Design review of the part built by this model. Coordinates are the model's own, in mm. A direction names the side the tool comes from. Round coordinates to 2 decimals unless told otherwise and drop trailing zeros. Order: outer loops, then holes, each group sorted by start corner. A loop starts at its lowest first (then second) coordinate and runs counter-clockwise, first axis right, second up. Notation, with made-up numbers: M 79,-27 L 90,-27 A22 cw 90,0 Z; hole C 3.5,20.25 d7. An arc over 180 degrees is marked long. Write item = value, one per line. Start each with the question number.
```python
from build123d import *

# Parameters (mm, degrees)
SKETCH2_R            = 15.24
BOSS_EXTRUDE1_DEPTH  = 5.08
SKETCH3_R            = 12.7
BOSS_EXTRUDE4_DEPTH  = 8.89
SKETCH4_R            = 7.62
SKETCH4_R_2          = 6.35
CUT_EXTRUDE2_DEPTH   = 0.508
SKETCH7_R            = 10.16
BOSS_EXTRUDE7_DEPTH  = 10.16
SKETCH8_R            = 6.35
SKETCH8_R_2          = 5.08
CUT_EXTRUDE6_DEPTH   = 1.27
SKETCH11_R           = 2.33542976
BOSS_EXTRUDE8_DEPTH  = 82.55
SKETCH12_R           = 6.35
BOSS_EXTRUDE9_DEPTH  = 2.54
SKETCH13_R           = 5.715
BOSS_EXTRUDE13_DEPTH = 1.905


with BuildPart() as part:
    # Sketch2 → Boss-Extrude1 (new body)
    with BuildSketch(Plane(origin=(0, 0, 0), x_dir=(1, 0, 0), z_dir=(0, 1, 0))):
        Circle(SKETCH2_R)
    extrude(amount=BOSS_EXTRUDE1_DEPTH)

    # Sketch3 → Boss-Extrude4 (add)
    with BuildSketch(Plane(origin=(0, 5.08, 0), x_dir=(1, 0, 0), z_dir=(0, 1, 0))):
        Circle(SKETCH3_R)
    extrude(amount=BOSS_EXTRUDE4_DEPTH)

    # Sketch4 → Cut-Extrude2 (cut)
    with BuildSketch(Plane(origin=(0, 13.97, 0), x_dir=(1, 0, 0), z_dir=(0, 1, 0))):
        Circle(SKETCH4_R)
        Circle(SKETCH4_R_2, mode=Mode.SUBTRACT)
    extrude(amount=-CUT_EXTRUDE2_DEPTH, mode=Mode.SUBTRACT)



with BuildPart() as body_2:
    # Sketch7 → Boss-Extrude7 (new body)
    with BuildSketch(Plane(origin=(0, 0, 0), x_dir=(1, 0, 0), z_dir=(0, 1, 0))):
        with Locations((0, -88.9)):
            Circle(SKETCH7_R)
    extrude(amount=BOSS_EXTRUDE7_DEPTH)

    # Sketch8 → Cut-Extrude6 (cut)
    with BuildSketch(Plane(origin=(0, 10.16, 0), x_dir=(1, 0, 0), z_dir=(0, 1, 0))):
        with Locations((0, -88.9)):
            Circle(SKETCH8_R)
        with Locations((0, -88.9)):
            Circle(SKETCH8_R_2, mode=Mode.SUBTRACT)
    extrude(amount=-CUT_EXTRUDE6_DEPTH, mode=Mode.SUBTRACT)


with BuildPart() as part_1:
    add(part.part)

    add(body_2.part)  # Boss-Extrude8 merges body 2
    # Sketch11 → Boss-Extrude8 (add)
    with BuildSketch(Plane.XY):
        with Locations((0, 2.324561436)):
            Circle(SKETCH11_R)
    extrude(amount=BOSS_EXTRUDE8_DEPTH)

    # Sketch12 → Boss-Extrude9 (add)
    with BuildSketch(Plane.XZ):
        with Locations((-0.225047318, 0)):
            Circle(SKETCH12_R)
    extrude(amount=BOSS_EXTRUDE9_DEPTH)

    # Sketch13 → Boss-Extrude13 (add)
    with BuildSketch(Plane.XZ):
        with Locations((0, 88.9)):
            Circle(SKETCH13_R)
    extrude(amount=BOSS_EXTRUDE13_DEPTH)


solid = part_1.part
```
(1) Insertion check: pin 1 (8 mm diameter, centred on x = -6.5, y = 9.5, fed in from -Z); pin 2 (5.5 mm diameter, centred on x = -1, z = 88, fed in from -Y) (3 decimals); pin 3 (4 mm diameter, centred on x = 2, z = 92, fed in from +Y). Each pin has a flat end and moves straight along its axis. Give the tip position at first contact, or say it passes through.
(2) Consider section B-B, the plane y = 6.75. Write out the cut boundary in (x, z).
(3) Draft analysis for pull direction Z (two halves, no side actions). For faces 1 (the face through (0, 10.16, 89)), 2 (the face through (-3.5, 5.08, -12.5)), state which applies: pulls with the +Z half, pulls with the -Z half, needs draft (parallel to the pull), parting line crosses it, or undercut.
(4) Consider section C-C, the plane z = 0. Write out the cut boundary in (x, y), then the cut area to 3 significant figures.
(5) For faces 3 (the face through (-2.75, 9.46, 12.4)), 4 (the face through (4.4, 0, 93.3)), 5 (the face through (1.078, 0.253, 52.377)), 6 (the face through (7, 10.16, 89)), 7 (the face through (0, -1.905, 89)), list the 3-axis set-ups (+Z, -Z, +X, -X, +Y, -Y) from which the entire face can be reached by the end or side of a thin tool; tool diameter is ignored.
(6) For line 1 along X through (y, z) = (13.75, 0); line 2 along Z through (x, y) = (0, 9.35), list the stretches that pass through material, from the lowest coordinate up. Write a range as [from, to].
(7) Consider section A-A, the plane z = 88.9. Write out the cut boundary in (x, y) (3 decimals), then the cut area to 3 significant figures.
(8) Consider section D-D, the plane y = 12.25. Write out the cut boundary in (x, z), then the cut area to 3 significant figures.
Completed:
q1.pin_1 = -12.45
q1.pin_2 = -1.905
q1.pin_3 = 10.16
q2.outline = C 0,0 d25.4; C 0,88.9 d20.32
q3.face_1 = needs draft
q3.face_2 = undercut
q4.outline = M -15.24,0 L -6.58,0 L -6.58,-2.54 L 6.12,-2.54 L 6.12,0 L 15.24,0 L 15.24,5.08 L 12.7,5.08 L 12.7,13.97 L 7.62,13.97 L 7.62,13.46 L 6.35,13.46 L 6.35,13.97 L -6.35,13.97 L -6.35,13.46 L -7.62,13.46 L -7.62,13.97 L -12.7,13.97 L -12.7,5.08 L -15.24,5.08 Z
q4.area = 412 mm2
q5.face_3 = +Y
q5.face_4 = -Y
q5.face_5 = none
q5.face_6 = +Z, +X, -X, +Y
q5.face_7 = +Z, +X, -X, -Y
q6.line_1 = [-12.7, -7.62], [-6.35, 6.35], [7.62, 12.7]
q6.line_2 = [-12.7, 12.7], [78.74, 82.55], [83.82, 93.98], [95.25, 99.06]
q7.outline = M -10.16,0 L -5.715,0 L -5.715,-1.905 L 5.715,-1.905 L 5.715,0 L 10.16,0 L 10.16,10.16 L 6.35,10.16 L 6.35,8.89 L 5.08,8.89 L 5.08,10.16 L -5.08,10.16 L -5.08,8.89 L -6.35,8.89 L -6.35,10.16 L -10.16,10.16 Z
q7.area = 225 mm2
q8.outline = C 0,0 d25.4
q8.area = 507 mm2
